Could you check a few things on this model? Use its own coordinates, in mm. Face numbers are marked on the shaded views. A direction names the side the tool comes from. Give positions to 0.01 mm unless a question says otherwise; leave off trailing zeros. Loops run counter-clockwise (first coordinate to the right, second up) from the corner with the lowest first, then second, coordinate; pieces in that order, holes last. Notation, with made-up numbers: M 84,85.5 L 139,85.5 A19 cw 139,119.5 Z; hole C 72,-25.5 d5. An arc over 180 degrees is marked long. Return JSON: item names as keys, results as strings. Group by question number.
1. For the marked faces 4, 5 and 6, which set-ups out of +Z, -Z, +X, -X, +Y, -Y let a thin tool reach every point of the face, with its end or its side?
2. For pin 1 (2 mm diameter, centred on x = 1135.5, z = 1062, fed in from +Y); pin 2 (6 mm diameter, centred on x = 338.5, z = 213, fed in from +Y); pin 3 (1 mm diameter, centred on x = 1103.5, y = -876.5, fed in from -Z), each with a flat end and sliding along its axis, tell me the tip position at first contact or that it passes through.
3. If we section it at C-C (y = -1120.5): Write out the boundary of the cut face in (x, z).
4. If we section it at B-B (x = 601): Write out the boundary of the cut face in (y, z), plus the area to 3 significant figures.
5. Please list where these lines run through material, in increasing order: line 1 (X direction, y = -953, z = 499); line 2 (Z direction, x = 894, y = -296); line 3 (Y direction, x = 582, z = 1014.5).
6. If we section it at D-D (z = 160.5): Write out the boundary of the cut face in (x, y), plus the area to 3 significant figures.
7. If we section it at A-A (z = 628): Write out the boundary of the cut face in (x, y), plus the area to 3 significant figures.
8. If we mould it in two halves opening along X, with no side actions, what happens to the marked faces 1, 2 and 3? For each: +X half, -X half, draft (parallel to the pull), parting line (faces both ways), or undercut.
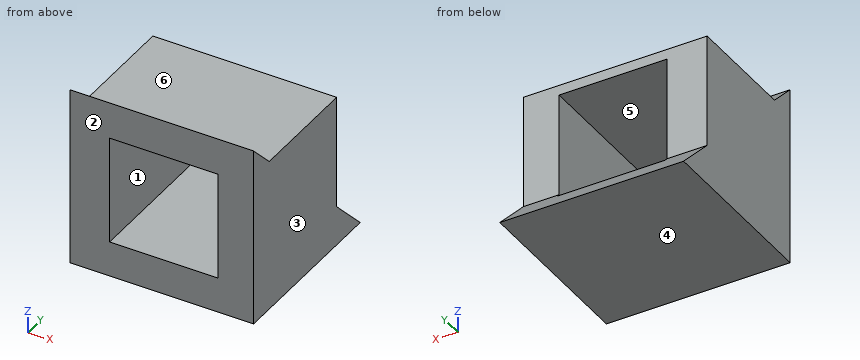
```python
from build123d import *

# Parameters (mm, degrees)
F0_W     = 1270
F0_H     = 1270
F0_W_2   = 762
F0_H_2   = 762
F1_DEPTH = 1270
F3_W     = 762
F3_H     = 762
F4_DEPTH = 12.7
F5_DEPTH = 1270.001
F6_DEPTH = 25.4


with BuildPart() as f1:
    # F0 (on Front) → F1 (new body)
    with BuildSketch(Plane.XZ):
        with Locations((635, 635)):
            Rectangle(F0_W, F0_H)
        with Locations((636.763900746, 631.1829624176)):
            Rectangle(F0_W_2, F0_H_2, mode=Mode.SUBTRACT)
    extrude(amount=F1_DEPTH)

    # F3 (on face) → F4 (cut, symmetric)
    with BuildSketch(Plane.XY.offset(1270)):
        with Locations((615.9371882677, -549.7496393476)):
            Rectangle(F3_W, F3_H)
    extrude(amount=F4_DEPTH, both=True, mode=Mode.SUBTRACT)

    # F2 (on face) → F5 (cut, through all)
    with BuildSketch(Plane.YZ.offset(1270)):
        Polygon((0, 1270), (-1270, 1270), (-1083.5376977921, 1083.5376977921), (-280.4070115089, 1083.5376977921), (-280.4070115089, 280.4070115089), (0, 0), align=None)
    extrude(amount=-F5_DEPTH, mode=Mode.SUBTRACT)

    # F6 (add): a face of the model
    f6_faces = [f1.faces().sort_by_distance(p)[0] for p in [
        (0, -761.3801568412, 535.4569952832),
    ]]
    extrude(f6_faces, amount=F6_DEPTH)


solid = f1.part
```
Answer:
{
 "1": {"face 4": "-Z, +X, -X, +Y, -Y", "face 5": "+Y, -Y", "face 6": "+Z, +X, -X, +Y"},
 "2": {"pin 1": "stops at y = -280.41", "pin 2": "stops at y = -210", "pin 3": "stops at z = 0"},
 "3": {"outline": "M -25.4,0 L 1270,0 L 1270,1120.5 L -25.4,1120.5 Z; hole M 255.76,250.18 L 1017.76,250.18 L 1017.76,1012.18 L 255.76,1012.18 Z"},
 "4": {"outline": "M -1270,0 L 0,0 L -250.18,250.18 L -1270,250.18 Z; M -1270,1012.18 L -280.41,1012.18 L -280.41,1083.54 L -1083.54,1083.54 L -1270,1270 Z", "area": "374,000 mm²"},
 "5": {"line 1": "x = -25.4 to 255.76, 1017.76 to 1270", "line 2": "z = 0 to 250.18, 1012.18 to 1083.54", "line 3": "y = -1270 to -280.41"},
 "6": {"outline": "M -25.4,-1270 L 1270,-1270 L 1270,-160.5 L -25.4,-160.5 Z", "area": "1,440,000 mm²"},
 "7": {"outline": "M -25.4,-1270 L 255.76,-1270 L 255.76,-280.41 L -25.4,-280.41 Z; M 1017.76,-1270 L 1270,-1270 L 1270,-280.41 L 1017.76,-280.41 Z", "area": "528,000 mm²"},
 "8": {"face 1": "undercut", "face 2": "draft", "face 3": "+X half"}
}
